```python
from build123d import *

# Parameters (mm, degrees)
F1_DEPTH      = 100
F1_DEPTH_BACK = 100
F2_R          = 1
F3_R          = 0.5


with BuildPart() as f1:
    # F0 (on Front) → F1 (new body, two sides)
    with BuildSketch(Plane.XZ) as f1_sk:
        with BuildLine():
            Line((-13.5, 7), (-13.5, -9))
            Line((-13.5, -9), (13.5, -9))
            Line((13.5, -9), (13.5, 7))
            ThreePointArc((13.5, 7), (11.5, 9), (9.5, 7))
            Line((9.5, 7), (10, 7))
            ThreePointArc((10, 7), (11.5, 8.5), (13, 7))
            Line((13, 7), (13, -8.5))
            Line((13, -8.5), (-13, -8.5))
            Line((-13, -8.5), (-13, 7))
            ThreePointArc((-13, 7), (-11.5, 8.5), (-10, 7))
            Line((-10, 7), (-9.5, 7))
            ThreePointArc((-9.5, 7), (-11.5, 9), (-13.5, 7))
        make_face()
    extrude(amount=F1_DEPTH)
    extrude(f1_sk.sketch, amount=-F1_DEPTH_BACK)

    # F2
    f2_edges = [f1.edges().sort_by_distance(p)[0] for p in [
        (13.5, 0, -9),
        (-13.5, 0, -9),
    ]]
    fillet(f2_edges, radius=F2_R)

    # F3
    f3_edges = [f1.edges().sort_by_distance(p)[0] for p in [
        (-13, 0, -8.5),
        (13, 0, -8.5),
    ]]
    fillet(f3_edges, radius=F3_R)


solid = f1.part
```
Source: CAD feature listing. Evaluate the final solid. Frame: model axes, mm. A direction names the side the tool comes from. Coordinates: 2 decimals unless noted, no trailing zeros. Order: outer loops, then holes, each group sorted by start corner. A loop starts at its lowest first (then second) coordinate and runs counter-clockwise, first axis right, second up. Notation, with made-up numbers: (-35.5, 34.25) - (22.5, 34.25) arc R30 ccw to (22.5, 73.25) - close; hole circle Ø8 at (-19, -12). An arc over 180 degrees is marked (long way). One line per item, written item: value.
1) Reachability of faces 4 (the face through (-13.5, -1, 0)), 5 (the face through (0, -1, -8.5)) from +Z, -Z, +X, -X, +Y, -Y: full face, straight path, thin tool, end or side. Return the list, or none.
Computed values:
face 4: +Z, -Z, -X, +Y, -Y
face 5: +Y, -Y
2) Cut plane A-A on z = 0.75. Output: boundary loops of the cut face in (x, y).
Computed values:
outline: (-13.5, -100) - (-13, -100) - (-13, 100) - (-13.5, 100) - close; (13, -100) - (13.5, -100) - (13.5, 100) - (13, 100) - close
3) Cut plane B-B on y = -77. Output: boundary loops of the cut face in (x, z), plus the area to 3 significant figures.
Computed values:
outline: (-13.5, -8) arc R1 ccw to (-12.5, -9) - (12.5, -9) arc R1 ccw to (13.5, -8) - (13.5, 7) arc R2 ccw to (9.5, 7) - (10, 7) arc R1.5 cw to (13, 7) - (13, -8) arc R0.5 cw to (12.5, -8.5) - (-12.5, -8.5) arc R0.5 cw to (-13, -8) - (-13, 7) arc R1.5 cw to (-10, 7) - (-9.5, 7) arc R2 ccw to (-13.5, 7) - close
area: 34.2 mm^2
4) Mould query, pull axis Z, two halves, no side actions, for faces 1 (the face through (13.5, -1, -1)), 2 (the face through (13, -1, 0)), 3 (the face through (-11.5, -1.4, 9)). Classes: released by +Z, released by -Z, zero draft, split by the parting line, or undercut.
Computed values:
face 1: zero draft
face 2: undercut
face 3: released by +Z
5) Contact query for a flat-ended pin moving along its axis: pin 1 (5 mm diameter, centred on x = -0.5, y = -59.5, fed in from +Z). Output: stop coordinate, or through.
Computed values:
pin 1: stops at z = -8.5
6) Cut plane C-C on x = -0.5. Output: boundary loops of the cut face in (y, z), plus the area to 3 significant figures.
Computed values:
outline: (-100, -9) - (100, -9) - (100, -8.5) - (-100, -8.5) - close
area: 100 mm^2
7) Ray query, line 1 (X direction, y = -84, z = -3.75); line 2 (X direction, y = 28.5, z = 7.5); line 3 (Z direction, x = -11.25, y = -73). Return the intervals inside material, ascending. Write a range as [from, to].
Computed values:
line 1: x = [-13.5, -13], [13, 13.5]
line 2: x = [-13.44, -12.91], [-10.09, -9.56], [9.56, 10.09], [12.91, 13.44]
line 3: z = [-9, -8.5], [8.48, 8.98]
